For this review, take the finished solid that the model builds, in its own axes (mm). Round coordinates to 2 decimals unless told otherwise and drop trailing zeros. Write each loop counter-clockwise with the first axis right and the second up, starting at its lowest first coordinate (ties: lowest second). Pieces come first, ordered by that corner, then holes. Notation, with made-up numbers: (66.25, 16) -> (72.25, 16) arc R26 ccw to (72.25, 36) -> close; hole circle Ø4 at (14, 58). An arc over 180 degrees is marked (long way). Write each question's results on one line, items separated by ' | '. Start each with the question number.
Item 1: Add section B-B (x = -1). State the section outline as (y, z) points, plus the area to 3 significant figures.
Item 2: Add section A-A (z = 1). State the section outline as (x, y) points, plus the area to 3 significant figures.
Item 3: To check wall thickness, follow line 1 along Z through (x, y) = (-4.75, -42.5); line 2 along X through (y, z) = (55.5, -6.5); line 3 along Z through (x, y) = (14, 128). State the ranges of each line that lie inside material, in increasing order.
Item 4: Clearance check with a flat-ended pin moving along its axis: pin 1 (3 mm diameter, centred on y = -40, z = 0.5, fed in from -X). State where the tip first meets the part, or that it passes through.
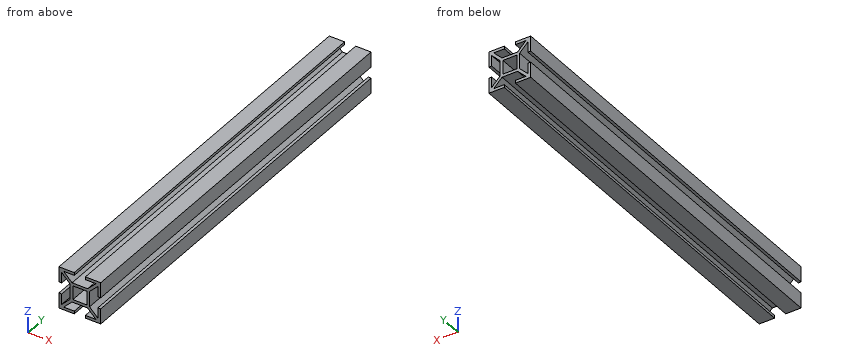
from build123d import *

# Parameters (mm, degrees)
F0_W     = 10
F0_H     = 10
F1_DEPTH = 145


with BuildPart() as f1:
    # F0 (on Front) → F1 (new body, symmetric)
    with BuildSketch(Plane.XZ):
        Polygon((7, -5.585787), (7, -7), (5.585787, -7), (11.585786, -13), (4, -13), (4, -15), (15, -15), (15, -4), (13, -4), (13, -11.585786), align=None)
        Polygon((5.585787, -7), (7, -7), (7, -5.585787), (7, 5.585787), (7, 7), (5.585787, 7), (-5.585787, 7), (-7, 7), (-7, 5.585787), (-7, -5.585787), (-7, -7), (-5.585787, -7), align=None)
        Rectangle(F0_W, F0_H, mode=Mode.SUBTRACT)
        Polygon((-11.585786, -13), (-5.585787, -7), (-7, -7), (-7, -5.585787), (-13, -11.585786), (-13, -4), (-15, -4), (-15, -15), (-4, -15), (-4, -13), align=None)
        Polygon((7, 7), (7, 5.585787), (13, 11.585786), (13, 4), (15, 4), (15, 15), (4, 15), (4, 13), (11.585786, 13), (5.585787, 7), align=None)
        Polygon((-13, 11.585786), (-7, 5.585787), (-7, 7), (-5.585787, 7), (-11.585786, 13), (-4, 13), (-4, 15), (-15, 15), (-15, 4), (-13, 4), align=None)
    extrude(amount=F1_DEPTH, both=True)


solid = f1.part
Responses:
1) outline: (-145, -7) -> (145, -7) -> (145, -5) -> (-145, -5) -> close; (-145, 5) -> (145, 5) -> (145, 7) -> (-145, 7) -> close | area: 1,160 mm^2
2) outline: (-7, -145) -> (-5, -145) -> (-5, 145) -> (-7, 145) -> close; (5, -145) -> (7, -145) -> (7, 145) -> (5, 145) -> close | area: 1,160 mm^2
3) line 1: z = -15 to -13, -7 to -5, 5 to 7, 13 to 15 | line 2: x = -15 to -13, -7.91 to 7.91, 13 to 15 | line 3: z = -15 to -4, 4 to 15
4) pin 1: stops at x = -7
